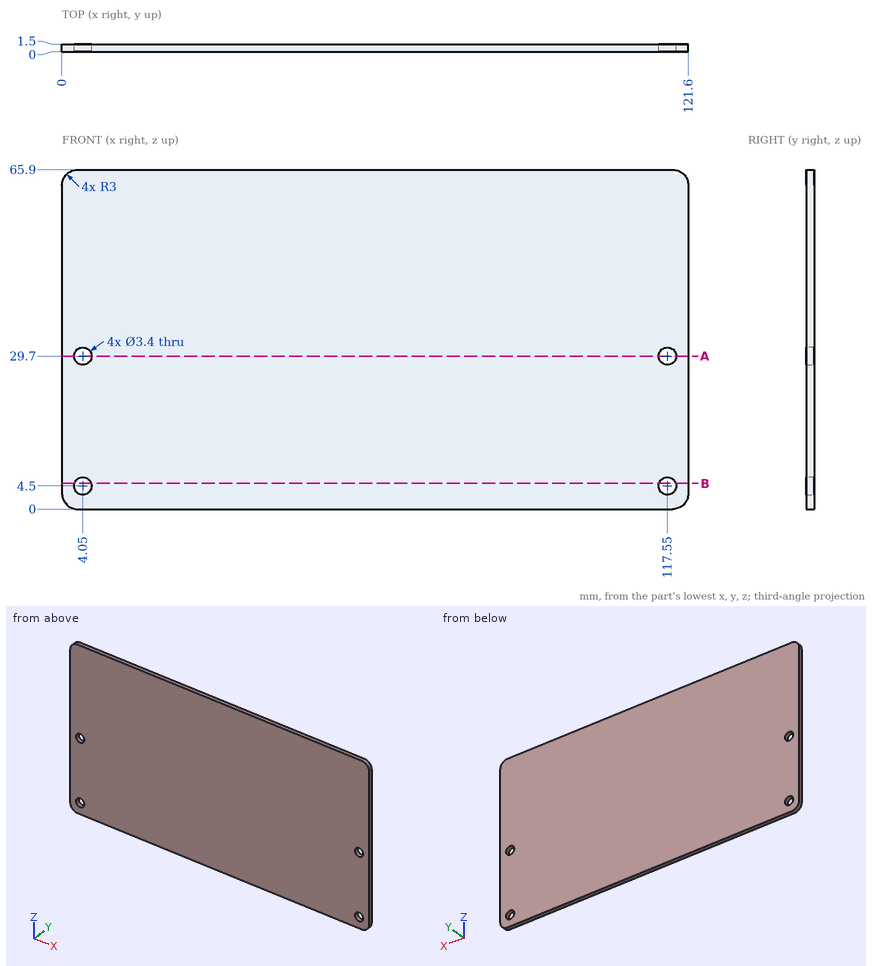
The figure shows three views and two pictorial views of one solid part (mm, origin at its lowest corner). Answer the questions. Round coordinates to 2 decimals unless told otherwise and drop trailing zeros. Write each loop counter-clockwise with the first axis right and the second up, starting at its lowest first coordinate (ties: lowest second). Pieces come first, ordered by that corner, then holes. Notation, with made-up numbers: (-4, 7) -> (54, 7) arc R27 cw to (54, 37) -> close; hole circle Ø10 at (-34.75, 34). An arc over 180 degrees is marked (long way). Answer as a JSON object with one key per item and string values. Group by question number.
Q1. Straight lines are drawn through the part: line 1 along X through (y, z) = (0.85, 29.7); line 2 along Z through (x, y) = (117.55, 1.25). For each, find the intervals that lie inside material, in ascending order.
Q2. Section B-B (z = 5) is taken. Write down the section's boundary in (x, y).
Q3. Section A-A (z = 29.7) is taken. Write down the section's boundary in (x, y).
Q4. This flat-tipped pin is pushed along its axis until it touches: pin 1 Ø2.5 at (x, z) = (4.05, 4.5) entering from -Y (3 decimals). Where does it stop, or does it pass through?
Check values:
{
 "1": {"line 1": "0 to 2.35, 5.75 to 115.85, 119.25 to 121.6", "line 2": "0 to 2.8, 6.2 to 28, 31.4 to 65.9"},
 "2": {"outline": "(0, 0) -> (2.43, 0) -> (2.43, 1.5) -> (0, 1.5) -> close; (5.67, 0) -> (115.93, 0) -> (115.93, 1.5) -> (5.67, 1.5) -> close; (119.17, 0) -> (121.6, 0) -> (121.6, 1.5) -> (119.17, 1.5) -> close"},
 "3": {"outline": "(0, 0) -> (2.35, 0) -> (2.35, 1.5) -> (0, 1.5) -> close; (5.75, 0) -> (115.85, 0) -> (115.85, 1.5) -> (5.75, 1.5) -> close; (119.25, 0) -> (121.6, 0) -> (121.6, 1.5) -> (119.25, 1.5) -> close"},
 "4": {"pin 1": "through"}
}
